Here's how the part is built. I have some questions about the finished solid (model axes, mm). A direction names the side the tool comes from. Coordinates: 2 decimals unless noted, no trailing zeros. Write each loop counter-clockwise with the first axis right and the second up, starting at its lowest first coordinate (ties: lowest second). Pieces come first, ordered by that corner, then holes. Notation, with made-up numbers: (6.5, 82) -> (43.5, 82) arc R24 ccw to (43.5, 107) -> close; hole circle Ø3 at (-6.5, 39). An arc over 180 degrees is marked (long way). Answer in a Markdown table with one row per item. Add a question column.
from build123d import *

# Parameters (mm, degrees)
F1_DEPTH = 150
F3_DEPTH = 163
F4_DEPTH = 145


with BuildPart() as f1:
    # F0 (on Front) → F1 (new body)
    with BuildSketch(Plane.XZ):
        Polygon((90.0722037068, 47.3391901924), (0.5319875367, 47.3391901924), (-89.0082286333, 47.3391901924), (-89.0082286333, 24.6384392554), (-12.9456477409, -0.1503442564), (0.5319875367, 26.651770349), (14.0096228144, -0.1503442564), (90.0722037068, 24.6384392554), align=None)
    extrude(amount=F1_DEPTH)

    # F2 (on Front) → F3 (cut)
    with BuildSketch(Plane.XZ):
        Polygon((-15.4821047033, 5.9351143447), (0.5319875367, 37.7813193113), (16.5460797768, 5.9351143447), (85.0722036495, 28.2677676632), (85.0722036495, 42.3391901351), (-84.008228576, 42.3391901351), (-84.008228576, 28.2677676632), align=None)
    extrude(amount=F3_DEPTH, mode=Mode.SUBTRACT)

    # F4 (cut): a face of the model
    f4_faces = [f1.faces().sort_by_distance(p)[0] for p in [
        (0.5319875367, -150, 29.1828717422),
    ]]
    extrude(f4_faces, amount=-F4_DEPTH, mode=Mode.SUBTRACT)


solid = f1.part
Q1. Imagine slicing it at C-C on z = 12.5. Please give me the cut outline in (x, y).
Q2. Imagine slicing it at B-B on x = -1. Please give me the cut outline in (y, z).
Q3. I need wall thicknesses on line 1 (X direction, y = -0.2, z = 38.5); line 2 (X direction, y = -4.2, z = 37.5); line 3 (Z direction, x = 25, y = -4). Which ranges of each line are inside material? Lowest first, please. Write a range as [from, to].
Q4. Imagine slicing it at D-D on x = -21.5. Please give me the cut outline in (y, z).
Q5. For faces 4 (the flat face through (7.176, -2.465, 13.438)), 5 (the flat face through (2, -2, 47.339)), 6 (the flat face through (8.427, -2.465, 22.081)), which set-ups out of +Z, -Z, +X, -X, +Y, -Y let a thin tool reach every point of the face, with its end or its side?
Q6. I'm going to push a flat-ended pin straight in: P1, Ø1.5, axis at x = 1, y = -3.5, coming from the -Z side. Where does the tip first touch, or does it pass through?
Q7. If we mould it in two halves opening along X, with no side actions, what happens to faces 1 (the flat face through (-7.587, -2.465, 21.635)), 2 (the flat face through (51.51, -2.46, 12.07)), 3 (the flat face through (0, -5, 29))? For each: pulls with the +X half, pulls with the -X half, needs draft (parallel to the pull), parting line crosses it, or undercut.
Q8. Imagine slicing it at A-A on y = -0.85. Please give me the cut outline in (x, z).
Result sheet:
| question | item | result |
|---|---|---|
| 1 | outline | (-51.76, -5) -> (-35.63, -5) -> (-35.63, 0) -> (-51.76, 0) -> close; (-12.18, -5) -> (-6.58, -5) -> (-6.58, 0) -> (-12.18, 0) -> close; (7.65, -5) -> (13.24, -5) -> (13.24, 0) -> (7.65, 0) -> close; (36.69, -5) -> (52.83, -5) -> (52.83, 0) -> (36.69, 0) -> close |
| 2 | outline | (-5, 23.61) -> (0, 23.61) -> (0, 34.73) -> (-5, 34.73) -> close; (-5, 42.34) -> (0, 42.34) -> (0, 47.34) -> (-5, 47.34) -> close |
| 3 | line 1 | x = [-89.01, -84.01], [85.07, 90.07] |
| 3 | line 2 | x = [-89.01, -84.01], [0.39, 0.67], [85.07, 90.07] |
| 3 | line 3 | z = [3.43, 8.69], [42.34, 47.34] |
| 4 | outline | (-5, 2.64) -> (0, 2.64) -> (0, 7.9) -> (-5, 7.9) -> close; (-5, 42.34) -> (0, 42.34) -> (0, 47.34) -> (-5, 47.34) -> close |
| 5 | face 4 | -Z, +Y, -Y |
| 5 | face 5 | +Z, +X, -X, +Y, -Y |
| 5 | face 6 | +Y, -Y |
| 6 | P1 | stops at z = 24.23 |
| 7 | face 1 | undercut |
| 7 | face 2 | pulls with the +X half |
| 7 | face 3 | needs draft |
| 8 | outline | (-89.01, 24.64) -> (-12.95, -0.15) -> (0.53, 26.65) -> (14.01, -0.15) -> (90.07, 24.64) -> (90.07, 47.34) -> (-89.01, 47.34) -> close; hole (-84.01, 28.27) -> (-15.48, 5.94) -> (0.53, 37.78) -> (16.55, 5.94) -> (85.07, 28.27) -> (85.07, 42.34) -> (-84.01, 42.34) -> close |
